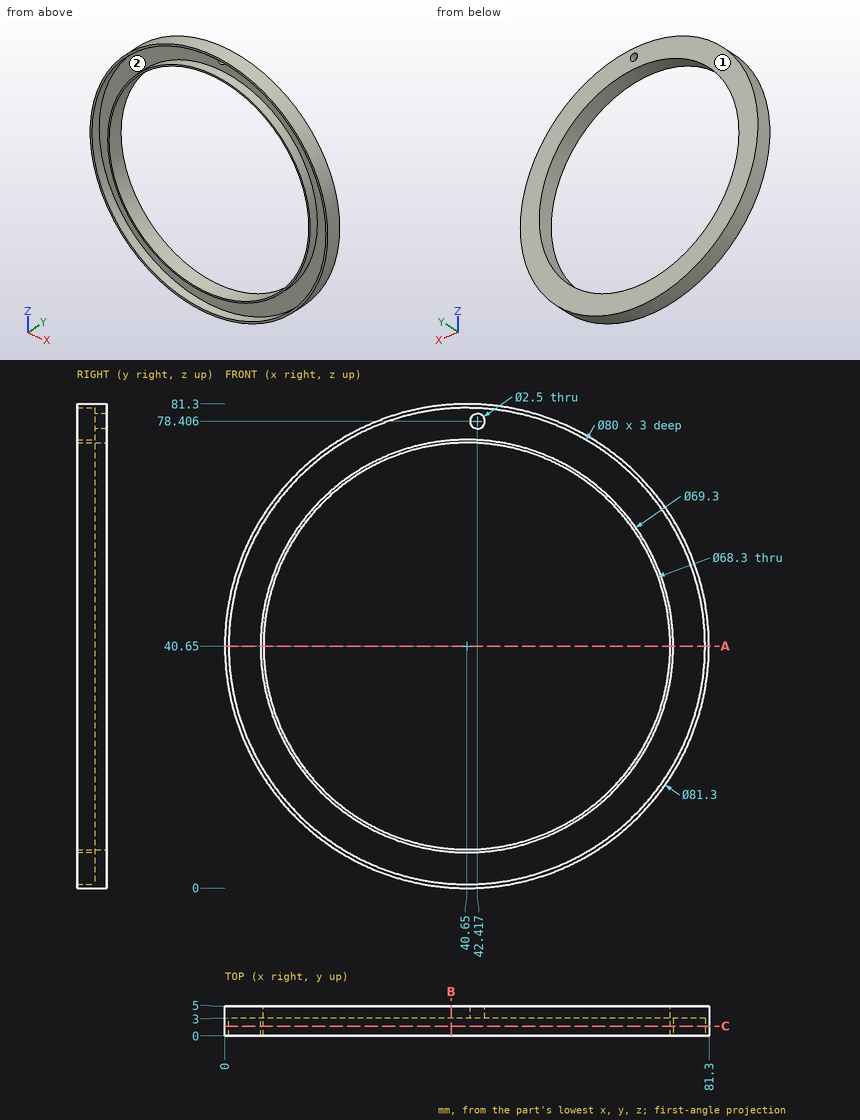
Study the drawing (mm; zero at the part's minimum x, y, z) and answer. Give positions to 0.01 mm unless a question says otherwise; leave off trailing zeros. Write each loop counter-clockwise with the first axis right and the second up, starting at its lowest first coordinate (ties: lowest second). Pieces come first, ordered by that corner, then holes.
(1) Straight lines are drawn through the part: line 1 (Z direction, x = 40.65, y = 2.6); line 2 (Z direction, x = 47.5, y = 2.4) (1 decimal); line 3 (Y direction, x = 76, z = 54). For each, find the intervals that lie inside material, in ascending order.
Final values:
line 1: z = 0 to 0.65, 6 to 6.5, 74.8 to 75.3, 80.65 to 81.3
line 2: z = 0.6 to 1.2, 6.7 to 7.2, 74.1 to 74.6, 80.1 to 80.7
line 3: y = 3 to 5
(2) A flat-ended cylindrical pin translates along its axis: pin 1 Ø24 at (x, z) = (48.5, 55) entering from -Y. Find the tip coordinate at first contact, or state that the pin passes through.
Final values:
pin 1: passes through
(3) The mould has two halves that part along X. Classify the marked faces 1 and 2: pulls with the +X half, pulls with the -X half, needs draft (parallel to the pull), parting line crosses it, or undercut.
Final values:
face 1: needs draft
face 2: undercut
(4) The part is cut by section A-A on z = 40.65. Write down the section's boundary in (x, y), plus the area to 3 significant figures.
Final values:
outline: (0, 0) - (0.65, 0) - (0.65, 3) - (6, 3) - (6, 0) - (6.5, 0) - (6.5, 5) - (0, 5) - close; (74.8, 0) - (75.3, 0) - (75.3, 3) - (80.65, 3) - (80.65, 0) - (81.3, 0) - (81.3, 5) - (74.8, 5) - close
area: 32.9 mm2
(5) The part is cut by section C-C on y = 1.65. Write down the section's boundary in (x, z).
Final values:
outline: circle Ø81.3 at (40.65, 40.65); circle Ø69.3 at (40.65, 40.65); hole circle Ø80 at (40.65, 40.65); hole circle Ø68.3 at (40.65, 40.65)
(6) The part is cut by section B-B on x = 38. Write down the section's boundary in (y, z).
Final values:
outline: (0, 0.09) - (5, 0.09) - (5, 6.6) - (0, 6.6) - (0, 6.1) - (3, 6.1) - (3, 0.74) - (0, 0.74) - close; (0, 74.7) - (5, 74.7) - (5, 81.21) - (0, 81.21) - (0, 80.56) - (3, 80.56) - (3, 75.2) - (0, 75.2) - close
